For this review, take the finished solid that the model builds, in its own axes (mm). A direction names the side the tool comes from. Give positions to 0.01 mm unless a question says otherwise; leave off trailing zeros. Write each loop counter-clockwise with the first axis right and the second up, starting at its lowest first coordinate (ties: lowest second). Pieces come first, ordered by that corner, then holes. Notation, with made-up numbers: M 10.5,88 L 29.5,88 A20 cw 29.5,126 Z; hole C -13.5,-26.75 d11. An arc over 180 degrees is marked long. Write item = value, one per line.
```python
from build123d import *

# Parameters (mm, degrees)
EXTRUDE1_REACH                 = 26.638
SKETCH13_W                     = 4.445
SKETCH13_H                     = 0.529166666
POINT_CUT_EXTRUDE10_DEPTH      = 7.096
POINT_CUT_EXTRUDE10_DEPTH_BACK = 7.096


with BuildPart() as part:
    # Sketch1 → base-Revolve (revolve)
    with BuildSketch(Plane.XY):
        Polygon((0, 6.096), (-0.762, 6.096), (-0.762, 4.6609), (-5.588, 4.6609), (-5.588, 3.72872), (-4.6228, 3.72872), (-4.6228, 0), (0, 0), (19.05, 0), (19.05, 3.175), (0, 3.175), align=None)
    revolve(axis=Axis((0, 0, 0), (1, 0, 0)))

    # Sketch15 → Extrude1 (add, up to next)
    with BuildSketch(Plane.ZY.offset(5.588), mode=Mode.PRIVATE) as extrude1_sk1:
        with BuildLine():
            ThreePointArc((-4.036457824, -2.330449967), (-4.6609, 3.6e-08), (-4.036457787, 2.33045003))
            Line((-4.036457787, 2.33045003), (-5.381943739, 0))
            Line((-5.381943739, 0), (-4.036457824, -2.330449967))
        make_face()
    extrude1_tool1 = extrude(extrude1_sk1.sketch, amount=-EXTRUDE1_REACH, mode=Mode.PRIVATE) - part.part
    add(extrude1_tool1.solids().sort_by_distance((-5.588, 0, -4.817334))[0])
    # Sketch15 → Extrude1 (add, up to next)
    with BuildSketch(Plane.ZY.offset(5.588), mode=Mode.PRIVATE) as extrude1_sk2:
        with BuildLine():
            ThreePointArc((-4.036457787, 2.33045003), (-2.330449985, 4.036457813), (0, 4.6609))
            Line((0, 4.6609), (-2.69097187, 4.6609))
            Line((-2.69097187, 4.6609), (-4.036457787, 2.33045003))
        make_face()
    extrude1_tool2 = extrude(extrude1_sk2.sketch, amount=-EXTRUDE1_REACH, mode=Mode.PRIVATE) - part.part
    add(extrude1_tool2.solids().sort_by_distance((-5.588, 4.171933, -2.408667))[0])
    # Sketch15 → Extrude1 (add, up to next)
    with BuildSketch(Plane.ZY.offset(5.588), mode=Mode.PRIVATE) as extrude1_sk3:
        with BuildLine():
            ThreePointArc((0, 4.6609), (2.330450001, 4.036457804), (4.036457805, 2.330449998))
            Line((4.036457805, 2.330449998), (2.69097187, 4.6609))
            Line((2.69097187, 4.6609), (0, 4.6609))
        make_face()
    extrude1_tool3 = extrude(extrude1_sk3.sketch, amount=-EXTRUDE1_REACH, mode=Mode.PRIVATE) - part.part
    add(extrude1_tool3.solids().sort_by_distance((-5.588, 4.171933, 2.408667))[0])
    # Sketch15 → Extrude1 (add, up to next)
    with BuildSketch(Plane.ZY.offset(5.588), mode=Mode.PRIVATE) as extrude1_sk4:
        with BuildLine():
            Line((4.036457776, -2.330450049), (5.381943739, 0))
            Line((5.381943739, 0), (4.036457805, 2.330449998))
            ThreePointArc((4.036457805, 2.330449998), (4.502083684, 1.206329686), (4.6609, 0))
            ThreePointArc((4.6609, 0), (4.502083676, -1.206329715), (4.036457776, -2.330450049))
        make_face()
    extrude1_tool4 = extrude(extrude1_sk4.sketch, amount=-EXTRUDE1_REACH, mode=Mode.PRIVATE) - part.part
    add(extrude1_tool4.solids().sort_by_distance((-5.588, 0, 4.817334))[0])
    # Sketch15 → Extrude1 (add, up to next)
    with BuildSketch(Plane.ZY.offset(5.588), mode=Mode.PRIVATE) as extrude1_sk5:
        with BuildLine():
            Line((2.69097187, -4.6609), (4.036457776, -2.330450049))
            ThreePointArc((4.036457776, -2.330450049), (2.330449975, -4.036457819), (0, -4.6609))
            Line((0, -4.6609), (2.69097187, -4.6609))
        make_face()
    extrude1_tool5 = extrude(extrude1_sk5.sketch, amount=-EXTRUDE1_REACH, mode=Mode.PRIVATE) - part.part
    add(extrude1_tool5.solids().sort_by_distance((-5.588, -4.171933, 2.408667))[0])
    # Sketch15 → Extrude1 (add, up to next)
    with BuildSketch(Plane.ZY.offset(5.588), mode=Mode.PRIVATE) as extrude1_sk6:
        with BuildLine():
            Line((-2.69097187, -4.6609), (0, -4.6609))
            ThreePointArc((0, -4.6609), (-2.330450017, -4.036457795), (-4.036457824, -2.330449967))
            Line((-4.036457824, -2.330449967), (-2.69097187, -4.6609))
        make_face()
    extrude1_tool6 = extrude(extrude1_sk6.sketch, amount=-EXTRUDE1_REACH, mode=Mode.PRIVATE) - part.part
    add(extrude1_tool6.solids().sort_by_distance((-5.588, -4.171933, -2.408667))[0])

    # Sketch8 → point_Cut-Revolve1 (revolve, cut)
    with BuildSketch(Plane.XY):
        Polygon((19.05, 0), (19.558, 0), (19.558, 3.683), (17.488209787, 3.683), (17.488209787, 3.175), (19.05, 2.2733), align=None)
    revolve(axis=Axis((0, 0, 0), (1, 0, 0)), mode=Mode.SUBTRACT)

    # Sketch13 → point_Cut-Extrude10 (cut, two sides)
    with BuildSketch(Plane.XY) as point_cut_extrude10_sk:
        with Locations((16.8275, 0)):
            Rectangle(SKETCH13_W, SKETCH13_H)
    extrude(amount=POINT_CUT_EXTRUDE10_DEPTH, mode=Mode.SUBTRACT)
    extrude(point_cut_extrude10_sk.sketch, amount=-POINT_CUT_EXTRUDE10_DEPTH_BACK, mode=Mode.SUBTRACT)


solid = part.part
```
1. We need section D-D, the plane y = -5. Write out the cut boundary in (x, z).
Responses:
outline = M -0.76,-3.49 L 0,-3.49 L 0,3.49 L -0.76,3.49 Z
2. For line 1 along X through (y, z) = (4.5, 0.5); line 2 along X through (y, z) = (-0.75, 3.25); line 3 along Y through (x, z) = (-2.75, 1), list the stretches that pass through material, from the lowest coordinate up. Write a range as from..to.
Responses:
line_1 = -5.59..0
line_2 = -4.62..0
line_3 = -4.66..4.66
3. Machinability: for faces 1 (the face through (-3, -4.661, 0)), 2 (the face through (-0.762, -3, -4)), 3 (the face through (-3, 4.661, 0)), which of the approach directions +Z, -Z, +X, -X, +Y, -Y give a long, thin tool a straight path to every point of the face, cutting with its end or side? Answer none if there is none.
Responses:
face_1 = +Z, -Z, -X, -Y
face_2 = -X
face_3 = +Z, -Z, -X, +Y
4. We need section C-C, the plane z = 0. Write out the cut boundary in (x, y) (3 decimals), then the cut area to 3 significant figures.
Responses:
outline = M -5.588,-4.661 L -0.762,-4.661 L -0.762,-6.096 L 0,-6.096 L 0,-3.175 L 17.488,-3.175 L 19.05,-2.273 L 19.05,-0.265 L 14.605,-0.265 L 14.605,0.265 L 19.05,0.265 L 19.05,2.273 L 17.488,3.175 L 0,3.175 L 0,6.096 L -0.762,6.096 L -0.762,4.661 L -5.588,4.661 L -5.588,3.729 L -4.623,3.729 L -4.623,-3.729 L -5.588,-3.729 Z
area = 164 mm2
5. The part is to be moulded in two halves that separate along Z. For faces 4 (the face through (8.62, -0.69, -3.1)), 5 (the face through (-5.1, -0.81, -3.64)), 6 (the face through (19.05, 1, 0)), say which applies: +Z half, -Z half, draft (parallel to the pull), parting line (faces both ways), or undercut.
Responses:
face_4 = parting line
face_5 = undercut
face_6 = draft
6. We need section A-A, the plane x = 15.75. Write out the cut boundary in (y, z) (3 decimals), then the cut area to 3 significant figures.
Responses:
outline = M -0.265,-3.164 L -0.265,3.164 A3.175 ccw Z; M 0.265,-3.164 A3.175 ccw 0.265,3.164 Z
area = 28.3 mm2
7. We need section B-B, the plane x = -2.5. Write out the cut boundary in (y, z), then the cut area to 3 significant figures.
Responses:
outline = M -4.66,-2.69 L 0,-5.38 L 4.66,-2.69 L 4.66,2.69 L 0,5.38 L -4.66,2.69 Z
area = 75.3 mm2
8. Insertion check: P1, Ø2, axis at x = 13, y = -3, coming from the -Z side; P2, Ø5.5, axis at x = -3, z = 1, coming from the -Y side; P3, Ø3, axis at x = 16, z = -0.5, coming from the -Y side (3 decimals); P4, Ø6.5, axis at y = 0, z = 0, coming from the -X side. Each pin has a flat end and moves straight along its axis. Give the tip position at first contact, or say it passes through.
Responses:
P1 = -2.47
P2 = -6.1
P3 = -3.175
P4 = -4.62
